Read the model definition and answer for the solid it produces. Units are mm, in the model's axes. Give positions to 0.01 mm unless a question says otherwise; leave off trailing zeros. Loops run counter-clockwise (first coordinate to the right, second up) from the corner with the lowest first, then second, coordinate; pieces in that order, holes last.
(1) Straight lines are drawn through the part: probe 1 along Z at (x, y) = (34, 25); probe 2 along Z at (x, y) = (4, 19); probe 3 along Y at (x, z) = (54, 31.5). For each, find the intervals that lie inside material, in ascending order.
(2) This flat-tipped pin is pushed along its axis until it touches: P1, Ø6, axis at x = 17.5, y = 35, coming from the -Z side. Where does it stop, or does it pass through?
(3) Find section C-C, the plane y = 8. Write down the section's boundary in (x, z).
(4) Find section B-B, the plane z = 38. Write down the section's boundary in (x, y), then the cut area to 3 significant figures.
(5) Find section D-D, the plane z = 12. Write down the section's boundary in (x, y), then the cut area to 3 significant figures.
(6) Find section A-A, the plane x = 34.5. Write down the section's boundary in (y, z).
```python
from build123d import *

# Parameters (mm, degrees)
SKETCH1_W           = 80
SKETCH1_H           = 60
BOSS_EXTRUDE1_DEPTH = 50
CUT_EXTRUDE1_DEPTH  = 50
CUT_EXTRUDE2_DEPTH  = 124
CUT_EXTRUDE3_DEPTH  = 124
CUT_EXTRUDE4_DEPTH  = 124
CUT_EXTRUDE5_DEPTH  = 124
CUT_EXTRUDE6_DEPTH  = 124
CUT_EXTRUDE7_DEPTH  = 124
CUT_EXTRUDE8_DEPTH  = 124
CUT_EXTRUDE9_DEPTH  = 124
CUT_EXTRUDE10_DEPTH = 124
CUT_EXTRUDE11_DEPTH = 124
CUT_EXTRUDE12_DEPTH = 124
CUT_EXTRUDE14_DEPTH = 124
CUT_EXTRUDE15_DEPTH = 124
BOSS_EXTRUDE2_DEPTH = 5
SKETCH27_W          = 80
SKETCH27_H          = 50
CUT_EXTRUDE20_DEPTH = 37


with BuildPart() as part:
    # Sketch1 → Boss-Extrude1 (new body)
    with BuildSketch(Plane.XY):
        with Locations((40, 30)):
            Rectangle(SKETCH1_W, SKETCH1_H)
    extrude(amount=BOSS_EXTRUDE1_DEPTH)

    # Sketch2 → Cut-Extrude1 (cut)
    with BuildSketch(Plane.XY.offset(50)):
        Polygon((0, 30), (20, 60), (0, 60), align=None)
    extrude(amount=-CUT_EXTRUDE1_DEPTH, mode=Mode.SUBTRACT)

    # Sketch3 → Cut-Extrude2 (cut)
    with BuildSketch(Plane(origin=(80, 0, 0), x_dir=(0, 0, -1), z_dir=(1, 0, 0))):
        Polygon((-30, 60), (-50, 40), (-50, 60), align=None)
    extrude(amount=-CUT_EXTRUDE2_DEPTH, mode=Mode.SUBTRACT)

    # Sketch6 → Cut-Extrude3 (cut)
    with BuildSketch(Plane(origin=(-15.714285714, 7.857142857, 23.571428571), x_dir=(0.845154255, 0.169030851, 0.507092553), z_dir=(-0.534522484, 0.267261242, 0.801783726))):
        Polygon((42.257712736, 47.434164903), (65.922031869, 22.135943621), (42.257712736, -15.811388301), align=None)
    extrude(amount=CUT_EXTRUDE3_DEPTH, mode=Mode.SUBTRACT)

    # Sketch7 → Cut-Extrude4 (cut)
    with BuildSketch(Plane(origin=(35.714285714, 7.142857143, 21.428571429), x_dir=(0.497245158, 0.099449032, -0.861891607), z_dir=(0.845154255, 0.169030851, 0.507092553))):
        Polygon((-33.149677207, 36.869833406), (-33.149677207, -3.922322703), (-9.944903162, 54.912517839), align=None)
    extrude(amount=-CUT_EXTRUDE4_DEPTH, mode=Mode.SUBTRACT)

    # Sketch8 → Cut-Extrude5 (cut)
    with BuildSketch(Plane(origin=(-16.483516484, -3.296703297, 28.571428571), x_dir=(-0.867610081, 0.056996283, -0.493967783), z_dir=(0.497245158, 0.099449032, -0.861891607))):
        Polygon((-25.736988098, 43.821678207), (-32.829858833, 45.467562834), (-42.05059079, 5.731205399), (-18.998760899, 4.408619538), (-18.998760899, 34.607663372), align=None)
    extrude(amount=-CUT_EXTRUDE5_DEPTH, mode=Mode.SUBTRACT)

    # Sketch9 → Cut-Extrude6 (cut)
    with BuildSketch(Plane(origin=(-22.751322751, 35.264550265, 26.164021164), x_dir=(0.887896271, 0.369460193, 0.274115627), z_dir=(0.460043706, -0.713067745, -0.529050262))):
        Polygon((32.208127825, 14.089089478), (39.138944356, 16.321024445), (48.149005846, -11.657874603), align=None)
    extrude(amount=-CUT_EXTRUDE6_DEPTH, mode=Mode.SUBTRACT)

    # Sketch10 → Cut-Extrude7 (cut)
    with BuildSketch(Plane(origin=(-0.962962963, -2.407407407, 2.407407407), x_dir=(0.962250449, -0.19245009, 0.19245009), z_dir=(0.272165527, 0.680413817, -0.680413817))):
        Polygon((8.581009883, -63.639610307), (7.076241761, -60.15846923), (13.471506281, -63.639610307), align=None)
    extrude(amount=-CUT_EXTRUDE7_DEPTH, mode=Mode.SUBTRACT)

    # Sketch11 → Cut-Extrude8 (cut)
    with BuildSketch(Plane(origin=(-15.346074938, 7.943850556, 1.805420581), x_dir=(-0.092282328, 0.047769676, -0.994586361), z_dir=(0.883262889, -0.457218437, -0.103913281))):
        Polygon((-47.510608217, 39.711812283), (-44.744502297, 37.117331923), (-48.456907611, 37.426149), (-48.456907611, 38.702914935), align=None)
    extrude(amount=-CUT_EXTRUDE8_DEPTH, mode=Mode.SUBTRACT)

    # Sketch12 → Cut-Extrude9 (cut)
    with BuildSketch(Plane(origin=(-7.230769231, 36.153846154, 0), x_dir=(0.980580676, 0.196116135, 0), z_dir=(0.196116135, -0.980580676, 0))):
        Polygon((13.335897189, 50), (13.830048081, 50), (13.335897189, 46.307692308), align=None)
    extrude(amount=-CUT_EXTRUDE9_DEPTH, mode=Mode.SUBTRACT)

    # Sketch15 → Cut-Extrude10 (cut)
    with BuildSketch(Plane(origin=(0, 50.769230769, 33.846153846), x_dir=(-1, 0, 0), z_dir=(0, -0.832050294, -0.554700196))):
        Polygon((-20, 16.641005887), (-80, 16.641005887), (-80, -19.414506868), (-40, -19.414506868), align=None)
    extrude(amount=-CUT_EXTRUDE10_DEPTH, mode=Mode.SUBTRACT)

    # Sketch16 → Cut-Extrude11 (cut)
    with BuildSketch(Plane(origin=(22.352941176, 6.877828054, -10.316742081), x_dir=(-0.385755922, -0.11869413, -0.914933917), z_dir=(0.874474632, 0.269069118, -0.403603676))):
        Polygon((-44.065195676, 50.107704244), (-33.13544456, 51.465023547), (-65.924697908, 26.467726395), align=None)
    extrude(amount=-CUT_EXTRUDE11_DEPTH, mode=Mode.SUBTRACT)

    # Sketch17 → Cut-Extrude12 (cut)
    with BuildSketch(Plane(origin=(-13.474892396, 53.122171946, 6.219181106), x_dir=(0.969698736, 0.242646617, 0.028407409), z_dir=(0.24430383, -0.96312087, -0.112755614))):
        Polygon((39.280526622, 22.819756729), (34.520919906, 12.887590849), (33.567164418, 22.827971688), (35.583149731, 23.962584818), align=None)
    extrude(amount=-CUT_EXTRUDE12_DEPTH, mode=Mode.SUBTRACT)

    # Sketch22 → Cut-Extrude14 (cut)
    with BuildSketch(Plane(origin=(-14.80441324, 9.869608826, 18.916750251), x_dir=(0.821599096, 0.263693024, 0.505411628), z_dir=(-0.57006572, 0.380043813, 0.728417309))):
        Polygon((42.361795907, 43.943770636), (72.790261699, 12.335093512), (40.333231521, -23.128300335), (18.019023273, 17.346225251), align=None)
    extrude(amount=CUT_EXTRUDE14_DEPTH, mode=Mode.SUBTRACT)

    # Sketch23 → Cut-Extrude15 (cut)
    with BuildSketch(Plane(origin=(17.379185671, 15.917127194, 5.296513728), x_dir=(0.161703891, 0.148100231, -0.97566294), z_dir=(0.719498347, 0.658969121, 0.219275687))):
        Polygon((-15.07025189, 22.123368133), (-22.755667886, 20.283347912), (-41.425957995, -7.45305002), align=None)
    extrude(amount=-CUT_EXTRUDE15_DEPTH, mode=Mode.SUBTRACT)

    # Sketch26 → Boss-Extrude2 (add)
    with BuildSketch(Plane(origin=(-14.80441324, 9.869608826, 18.916750251), x_dir=(0.821599096, 0.263693024, 0.505411628), z_dir=(-0.57006572, 0.380043813, 0.728417309))):
        Polygon((18.019023273, -16.491483717), (40.333231521, -23.128300335), (72.790261699, 12.335093512), (42.361795907, 43.943770636), (18.019023273, 17.346225251), align=None)
    extrude(amount=-BOSS_EXTRUDE2_DEPTH)

    # Sketch27 → Cut-Extrude20 (cut)
    with BuildSketch(Plane.XZ):
        with Locations((40, 25)):
            Rectangle(SKETCH27_W, SKETCH27_H)
    extrude(amount=CUT_EXTRUDE20_DEPTH, mode=Mode.SUBTRACT)


solid = part.part
```
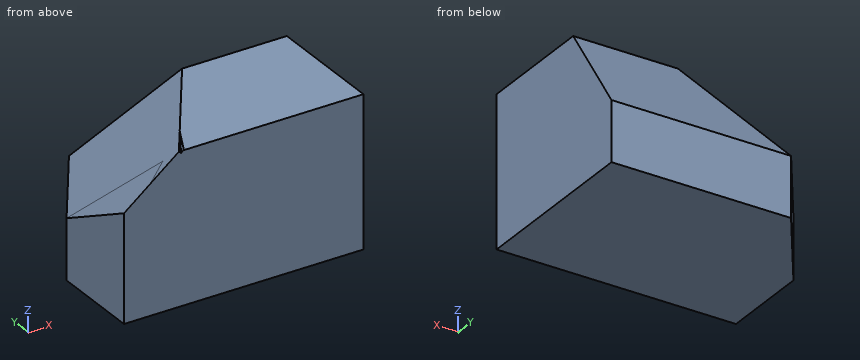
Entries:
1. probe 1: z = 0 to 49.22
1. probe 2: z = 0 to 28.87
1. probe 3: y = 0 to 52.33
2. P1: stops at z = 0
3. outline: (0, 0) - (80, 0) - (80, 50) - (24, 50) - (23.81, 49.87) - (23.67, 50) - (0, 31.48) - close
4. outline: (3, 0) - (80, 0) - (80, 48) - (35, 48) - close
4. area: 2,930 mm2
5. outline: (0, 0) - (80, 0) - (80, 60) - (20, 60) - (0, 30) - close
5. area: 4,500 mm2
6. outline: (0, 0) - (60, 0) - (60, 20) - (48.4, 37.4) - (24.25, 50) - (0, 50) - close
